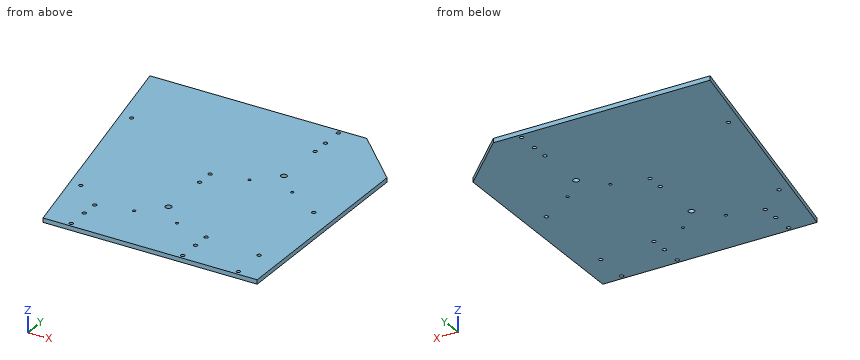
Autodesk Inventor part; units mm, degrees
ref_plane "YZ Plane" through (0, 0, 0) normal (1, 0, 0) x (0, 1, 0)
ref_plane "XZ Plane" through (0, 0, 0) normal (0, 1, 0) x (-1, 0, 0)
ref_plane "XY Plane" through (0, 0, 0) normal (0, 0, 1) x (1, 0, 0)
sketch "Sketch1" plane through (0, 0, 0) normal (0, 0, 1) x (1, 0, 0)
  line L0 (0, 0) -> (-63.0702, 310)
  line L1 (-63.0702, 310) -> (250, 310)
  line L2 (250, 310) -> (250, 0)
  line L3 (250, 0) -> (0, 0)
  dimension "d0" = 310
  dimension "d1" = 78.5
  dimension "d2" = 250
extrude "Extrusion1" add sketch "Sketch1" along normal blind 5
sketch "Sketch2" plane through (0, 0, 5) normal (0, 0, 1) x (1, 0, 0)
  line L0 (0, 0) -> (250, 0)
  point P0 (160, 280)
  point P1 (160, 260)
  point P2 (95, 165)
  point P3 (95, 145)
  point P4 (225, 150)
  point P5 (225, 45)
  point P6 (30, 50)
  point P7 (30, 30)
  point P8 (160, 50)
  point P9 (160, 30)
  point P10 (160, 305)
  point P11 (30, 5)
  point P12 (160, 5)
  point P13 (225, 5)
  dimension "d7" = 20
  dimension "d15" = 25
  dimension "d20" = 5
  dimension "d21" = 30
  dimension "d30" = 130
  dimension "d32" = 65
  dimension "d36" = 65
  dimension "d92" = 25
  dimension "d93" = 20
  dimension "d94" = 95
  dimension "d95" = 20
  dimension "d96" = 95
  dimension "d97" = 105
  dimension "d98" = 130
  dimension "d99" = 15
hole "Hole1" at (160, 280, 5) at (160, 260, 5) at (95, 165, 5) at (95, 145, 5) at (225, 150, 5) at (225, 45, 5) at (30, 50, 5) at (30, 30, 5) at (160, 50, 5) at (160, 30, 5) at (160, 305, 5) at (30, 5, 5) at (160, 5, 5) at (225, 5, 5) direction (0, 0, -1) diameter 4.5 end through all
sketch "Sketch3" plane through (0, 0, 5) normal (0, 0, 1) x (1, 0, 0)
  circle A0 centre (30, 5) radius 2.25
  circle A1 centre (160, 30) radius 2.25
  circle A2 centre (30, 30) radius 2.25
  circle A3 centre (225, 45) radius 2.25
  circle A4 centre (95, 145) radius 2.25
  circle A5 centre (160, 260) radius 2.25
  circle A6 centre (160, 280) radius 2.25
  circle A7 centre (95, 165) radius 2.25
  circle A8 centre (225, 150) radius 2.25
  circle A9 centre (30, 50) radius 2.25
  circle A10 centre (160, 50) radius 2.25
  circle A11 centre (160, 5) radius 2.25
  line L0 (-63.0702, 310) -> (0, 0)
  line L1 (0, 0) -> (250, 0)
  line L2 (250, 0) -> (250, 310)
  line L3 (250, 310) -> (-63.0702, 310)
  point P0 (160, 200)
  point P1 (95, 85)
  dimension "d37" = 60
  dimension "d89" = 60
hole "Hole2" at (160, 200, 5) at (95, 85, 5) direction (0, 0, -1) diameter 7 end through all
sketch "Sketch4" plane through (0, 0, 5) normal (0, 0, 1) x (1, 0, 0)
  circle A0 centre (95, 85) radius 3.5
  circle A1 centre (160, 200) radius 3.5
  circle A2 centre (30, 5) radius 2.25
  circle A3 centre (160, 30) radius 2.25
  circle A4 centre (30, 30) radius 2.25
  circle A5 centre (225, 45) radius 2.25
  circle A6 centre (95, 145) radius 2.25
  circle A7 centre (160, 260) radius 2.25
  circle A8 centre (160, 280) radius 2.25
  circle A9 centre (95, 165) radius 2.25
  circle A10 centre (225, 150) radius 2.25
  circle A11 centre (30, 50) radius 2.25
  circle A12 centre (160, 50) radius 2.25
  circle A13 centre (160, 5) radius 2.25
  line L0 (-63.0702, 310) -> (0, 0)
  line L1 (0, 0) -> (250, 0)
  line L2 (250, 0) -> (250, 310)
  line L3 (250, 310) -> (-63.0702, 310)
  point P0 (185, 175)
  point P1 (135, 175)
  point P2 (70, 60)
  point P3 (120, 60)
  dimension "d46" = 25
  dimension "d47" = 25
  dimension "d48" = 50
  dimension "d49" = 50
  dimension "d50" = 25
hole "Hole3" at (185, 175, 5) at (135, 175, 5) at (70, 60, 5) at (120, 60, 5) direction (0, 0, -1) diameter 3.4 end through all
chamfer "Chamfer1" distance 60 angle 45 1 edges at (250, 310, 2.5)
sketch "Sketch5" plane through (0, 0, 5) normal (0, 0, 1) x (1, 0, 0)
  line L0 (-63.0702, 310) -> (0, 0)
  line L1 (190, 310) -> (-63.0702, 310)
  line L2 (0, 0) -> (250, 0)
  point P0 (-33.0207, 225)
  point P1 (-3.1155, 78.0113)
  dimension "d64" = 12.5
  dimension "d65" = 12.5
  dimension "d66" = 150
  dimension "d67" = 85
  dimension "d68" = 78.0113
hole "Hole4" at (-33.0207, 225, 5) at (-3.1155, 78.0113, 5) direction (0, 0, -1) diameter 4.5 end through all
sketch "Sketch6" plane through (0, 0, 5) normal (0, 0, 1) x (1, 0, 0)
  circle A0 centre (-33.0207, 225) radius 2.25
  circle A1 centre (-3.1155, 78.0113) radius 2.25
  line L0 (190, 310) -> (250, 250)
  line L1 (190, 310) -> (-63.0702, 310)
  line L2 (-63.0702, 310) -> (0, 0)
  line L3 (0, 0) -> (250, 0)
  line L4 (250, 0) -> (250, 250)
  circle A2 centre (70, 60) radius 1.7
  circle A3 centre (185, 175) radius 1.7
  circle A4 centre (135, 175) radius 1.7
  circle A5 centre (120, 60) radius 1.7
  circle A6 centre (95, 85) radius 3.5
  circle A7 centre (160, 200) radius 3.5
  circle A8 centre (30, 5) radius 2.25
  circle A9 centre (160, 30) radius 2.25
  circle A10 centre (30, 30) radius 2.25
  circle A11 centre (225, 45) radius 2.25
  circle A12 centre (95, 145) radius 2.25
  circle A13 centre (95, 165) radius 2.25
  circle A14 centre (225, 150) radius 2.25
  circle A15 centre (30, 50) radius 2.25
  circle A16 centre (160, 50) radius 2.25
  circle A17 centre (160, 5) radius 2.25
  point P0 (95.4041, 170)
  point P1 (115, 174)
  point P2 (205, 174)
  point P3 (224.5959, 170)
  dimension "d76" = 20
  dimension "d77" = 4
  dimension "d78" = 20
  dimension "d79" = 45
  dimension "d80" = 26
  dimension "d81" = 45
hole "Hole5" [suppressed]
equation "\"d5\" = d6"
properties part number "Top_Separator Backboard 3 Lanes" material "PMMA Plastic"
Read the model definition and answer for the solid it produces. Units are mm, in the model's axes. Give positions to 0.01 mm unless a question says otherwise; leave off trailing zeros. Write each loop counter-clockwise with the first axis right and the second up, starting at its lowest first coordinate (ties: lowest second). Pieces come first, ordered by that corner, then holes. Notation, with made-up numbers: (35, 1) - (57, 1) arc R26 cw to (57, 15) - close; hole circle Ø7 at (85, -18). An arc over 180 degrees is marked (long way). Answer in a Markdown table with one row per item. Add a question column.
Item 1: Section B-B, the plane x = -40 is taken. Write down the section's boundary in (y, z), and give its area (3 significant figures).
Item 2: Section A-A, the plane z = 3 is taken. Count the separate pieces of the cut face and the enclosed holes in it, and give its area (3 significant figures).
Item 3: Section C-C, the plane y = 234.5 is taken. Write down the section's boundary in (x, z).
Item 4: Find the intervals of material crossed by L1, parallel to Y at x = 30, z = 4.7; L2, parallel to Y at x = 226, z = 2.85; L3, parallel to X at y = 29, z = 1.55, in increasing order.
Item 5: A flat-ended cylindrical pin translates along its axis: P1, Ø1.5, axis at y = 261, z = 2.5, coming from the +X side. Find the tip coordinate at first contact, or state that the pin passes through.
Recorded:
| question | item | result |
|---|---|---|
| 1 | outline | (196.61, 0) - (310, 0) - (310, 5) - (196.61, 5) - close |
| 1 | area | 567 mm2 |
| 2 | separate pieces | 1 |
| 2 | enclosed holes | 22 |
| 2 | area | 85,100 mm2 |
| 3 | outline | (-47.71, 0) - (250, 0) - (250, 5) - (-47.71, 5) - close |
| 4 | L1 | y = 0 to 2.75, 7.25 to 27.75, 32.25 to 47.75, 52.25 to 310 |
| 4 | L2 | y = 0 to 2.98, 7.02 to 42.98, 47.02 to 147.98, 152.02 to 274 |
| 4 | L3 | x = -5.9 to 27.98, 32.02 to 157.98, 162.02 to 250 |
| 5 | P1 | stops at x = 239.75 |
